The figure shows three views and two pictorial views of one solid part (mm, origin at its lowest corner). Answer the questions. A direction names the side the tool comes from. Coordinates: 2 decimals unless noted, no trailing zeros. Write each loop counter-clockwise with the first axis right and the second up, starting at its lowest first coordinate (ties: lowest second). Pieces come first, ordered by that corner, then holes.
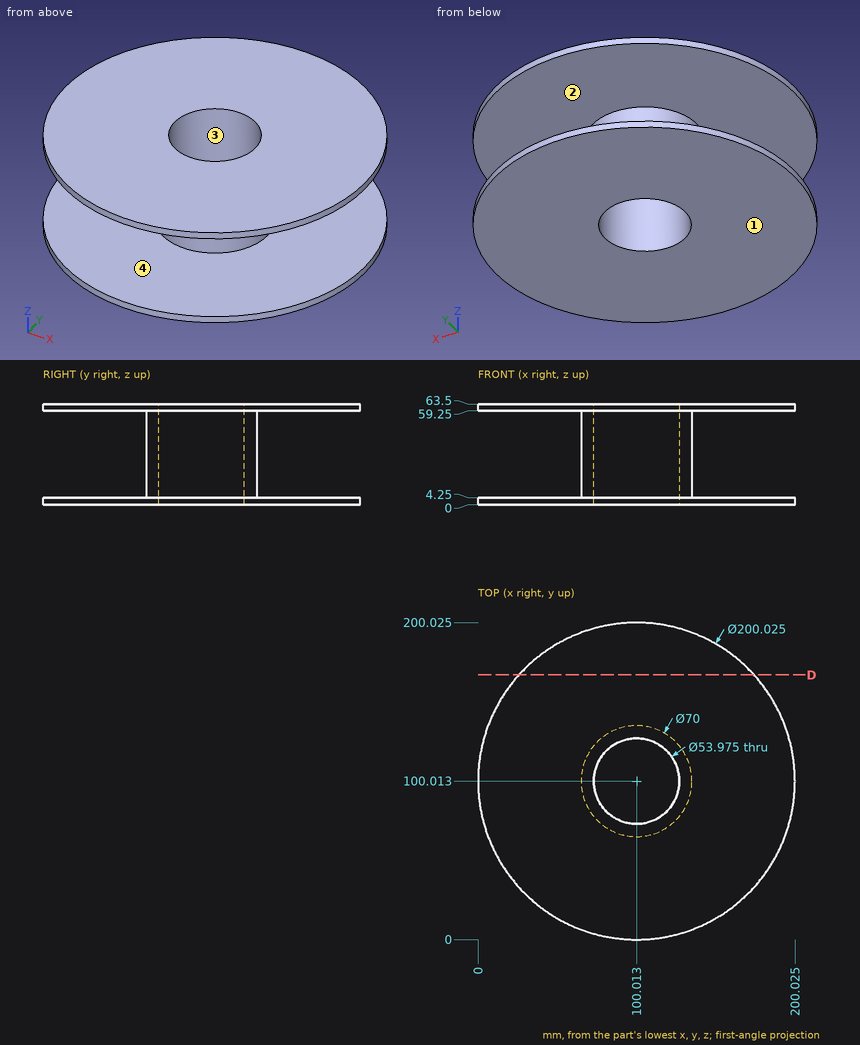
1. Section D-D on y = 167 is taken. Give the vertices of the cut face in (x, z).
Results found:
outline: (25.75, 0) - (174.28, 0) - (174.28, 4.25) - (25.75, 4.25) - close; (25.75, 59.25) - (174.28, 59.25) - (174.28, 63.5) - (25.75, 63.5) - close
2. For a pull along X with two mould halves and no side action, classify the marked faces 3 and 4 as pulls with the +X half, pulls with the -X half, needs draft (parallel to the pull), parting line crosses it, or undercut.
Results found:
face 3: undercut
face 4: needs draft
3. A tool of negligible diameter and unlimited length cuts with its end or side. For the marked faces 1 and 2, from which of +Z, -Z, +X, -X, +Y, -Y can it reach the whole face along a straight path? Write none if from no direction.
Results found:
face 1: -Z, +X, -X, +Y, -Y
face 2: none
4. Find the intervals of material crossed by L1, parallel to Z at x = 130, y = 133; L2, parallel to X at y = 106.5, z = 10 (1 decimal); L3, parallel to X at y = 90.5, z = 59 (1 decimal), in increasing order.
Results found:
L1: z = 0 to 4.25, 59.25 to 63.5
L2: x = 65.6 to 73.8, 126.2 to 134.4
L3: x = 66.3 to 74.8, 125.3 to 133.7
5. A flat-ended cylindrical pin translates along its axis: P1, Ø8, axis at x = 122.5, z = 35.5, coming from the -Y side (1 decimal). Find the tip coordinate at first contact, or state that the pin passes through.
Results found:
P1: stops at y = 70.3
